from build123d import *

# Parameters (mm, degrees)
SKETCH1_W           = 45
SKETCH1_H           = 24
BOSS_EXTRUDE1_DEPTH = 1.5
FILLET1_R           = 1
CUT_EXTRUDE1_REACH  = 27.544
SKETCH2_R           = 1.5


with BuildPart() as part:
    # Sketch1 → Boss-Extrude1 (new body)
    with BuildSketch(Plane(origin=(0, 0, 0), x_dir=(1, 0, 0), z_dir=(0, 1, 0))):
        Rectangle(SKETCH1_W, SKETCH1_H)
    extrude(amount=BOSS_EXTRUDE1_DEPTH)

    # Fillet1
    fillet1_edges = [part.edges().sort_by_distance(p)[0] for p in [
        (22.5, 0.75, 12),
        (-22.5, 0.75, 12),
        (-22.5, 0.75, -12),
        (22.5, 0.75, -12),
    ]]
    fillet(fillet1_edges, radius=FILLET1_R)

    # Sketch2 → Cut-Extrude1 (cut, up to next)
    with BuildSketch(Plane(origin=(0, 1.5, 0), x_dir=(1, 0, 0), z_dir=(0, 1, 0)), mode=Mode.PRIVATE) as cut_extrude1_sk1:
        with Locations(Location((-14, 0, 0), (0, 0, 270))):
            Circle(SKETCH2_R)
    cut_extrude1_tool1 = extrude(cut_extrude1_sk1.sketch, amount=-CUT_EXTRUDE1_REACH, mode=Mode.PRIVATE) & part.part
    # Sketch2 → Cut-Extrude1 (cut, up to next)
    with BuildSketch(Plane(origin=(0, 1.5, 0), x_dir=(1, 0, 0), z_dir=(0, 1, 0)), mode=Mode.PRIVATE) as cut_extrude1_sk2:
        with Locations(Location((14, 0, 0), (0, 0, 90))):
            Circle(SKETCH2_R)
    cut_extrude1_tool2 = extrude(cut_extrude1_sk2.sketch, amount=-CUT_EXTRUDE1_REACH, mode=Mode.PRIVATE) & part.part
    add(cut_extrude1_tool1.solids().sort_by_distance((-14, 1.5, 0))[0], mode=Mode.SUBTRACT)
    add(cut_extrude1_tool2.solids().sort_by_distance((14, 1.5, 0))[0], mode=Mode.SUBTRACT)


solid = part.part
CAD build for the part. Positions are in the model's coordinates, mm. Round coordinates to 2 decimals unless told otherwise and drop trailing zeros. Write each loop counter-clockwise with the first axis right and the second up, starting at its lowest first coordinate (ties: lowest second). Pieces come first, ordered by that corner, then holes.
(1) Mould opens along X. For faces 1 (the face through (0, 1, -12)), 2 (the face through (22.215, 0.76, -11.699)), 3 (the face through (-13.55, 0.76, 1.43)), 4 (the face through (-22.215, 0.76, 11.699)) say: pulls with the +X half, pulls with the -X half, needs draft (parallel to the pull), parting line crosses it, or undercut.
(2) Probe line 1 along X through (y, z) = (0.85, 0); line 2 along Z through (x, y) = (14, 0.6); line 3 along X through (y, z) = (0.8, -1). List the from-to ranges inside material, lowest first.
(3) Slice it at B-B, the plane z = 0. Write the cut outline in (x, y), and give its area (3 significant figures).
(4) Slice it at A-A, the plane x = -14. Write the cut outline in (y, z).
From the geometry:
1. face 1: needs draft
1. face 2: pulls with the +X half
1. face 3: undercut
1. face 4: pulls with the -X half
2. line 1: x = -22.5 to -15.5, -12.5 to 12.5, 15.5 to 22.5
2. line 2: z = -12 to -1.5, 1.5 to 12
2. line 3: x = -22.5 to -15.12, -12.88 to 12.88, 15.12 to 22.5
3. outline: (-22.5, 0) - (-15.5, 0) - (-15.5, 1.5) - (-22.5, 1.5) - close; (-12.5, 0) - (12.5, 0) - (12.5, 1.5) - (-12.5, 1.5) - close; (15.5, 0) - (22.5, 0) - (22.5, 1.5) - (15.5, 1.5) - close
3. area: 58.5 mm2
4. outline: (0, -12) - (1.5, -12) - (1.5, -1.5) - (0, -1.5) - close; (0, 1.5) - (1.5, 1.5) - (1.5, 12) - (0, 12) - close
